Read the model definition and answer for the solid it produces. Units are mm, in the model's axes. Face numbers are marked on the shaded views. A direction names the side the tool comes from. Round coordinates to 2 decimals unless told otherwise and drop trailing zeros. Order: outer loops, then holes, each group sorted by start corner. A loop starts at its lowest first (then second) coordinate and runs counter-clockwise, first axis right, second up. Notation, with made-up numbers: (42, 9) - (59, 9) arc R30 cw to (59, 32) - close; hole circle Ø6 at (-12.5, 55). An arc over 180 degrees is marked (long way). One line per question, with ' | ' between items. Start each with the question number.
1) The part is cut by section C-C, the plane z = -73. Give the vertices of the cut face in (x, y), plus the area to 3 significant figures.
2) Flat-ended cylindrical pins translate along their axes: pin 1 (8 mm diameter, centred on x = 37.5, z = 50.5, fed in from +Y); pin 2 (8 mm diameter, centred on y = 7, z = 38, fed in from +X); pin 3 (6 mm diameter, centred on x = 46, y = 7, fed in from -Z); pin 4 (5 mm diameter, centred on x = 73, z = 0, fed in from -Y). Find the tip coordinate at first contact, or state that the pin passes through.
3) The mould has two halves that part along X. Classify the marked faces 1, 2 and 3: pulls with the +X half, pulls with the -X half, needs draft (parallel to the pull), parting line crosses it, or undercut.
4) The part is cut by section B-B, the plane y = 29.5. Give the vertices of the cut face in (x, z), plus the area to 3 significant figures.
5) The part is cut by section A-A, the plane x = 0. Give the vertices of the cut face in (y, z).
6) The part is cut by section D-D, the plane x = -73. Give the vertices of the cut face in (y, z), plus the area to 3 significant figures.
7) Straight lines are drawn through the part: line 1 (X direction, y = 44, z = 0); line 2 (Y direction, x = 12.5, z = -52). For each, find the intervals that lie inside material, in ascending order. Write a range as from..to.
8) For the marked faces 4 and 5, determine the directions among +Z, -Z, +X, -X, +Y, -Y from which every point of the face is accessible in a straight line to the end or side of a thin tool.
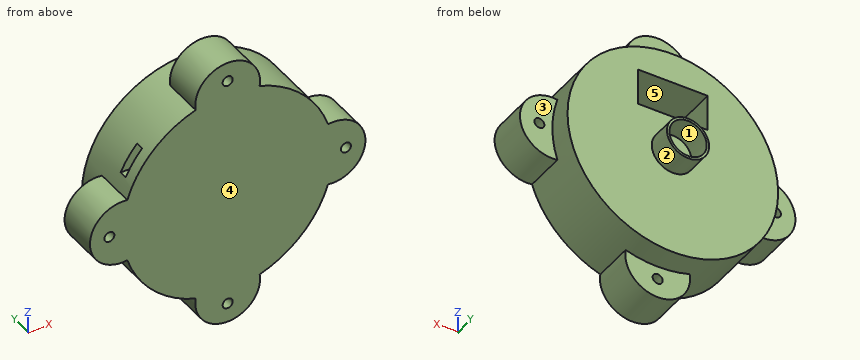
from build123d import *

# Parameters (mm, degrees)
SKETCH2_R           = 65
BOSS_EXTRUDE1_DEPTH = 40
SKETCH4_W           = 43
SKETCH4_H           = 22.5
CUT_EXTRUDE1_DEPTH  = 38
SKETCH6_R           = 3.1
BOSS_EXTRUDE2_DEPTH = 25
SKETCH9_R           = 13
SKETCH9_R_2         = 11.5
BOSS_EXTRUDE3_DEPTH = 15
SKETCH5_W           = 15
SKETCH5_H           = 5
CUT_EXTRUDE2_DEPTH  = 60


with BuildPart() as part:
    # Sketch2 → Boss-Extrude1 (new body)
    with BuildSketch(Plane(origin=(0, 0, 0), x_dir=(1, 0, 0), z_dir=(0, 1, 0))):
        Circle(SKETCH2_R)
    extrude(amount=BOSS_EXTRUDE1_DEPTH)

    # Sketch4 → Cut-Extrude1 (cut)
    with BuildSketch(Plane.XZ.offset(-40)):
        with Locations((0, 35)):
            Rectangle(SKETCH4_W, SKETCH4_H)
    extrude(amount=CUT_EXTRUDE1_DEPTH, mode=Mode.SUBTRACT)

    # Sketch6 → Boss-Extrude2 (add)
    with BuildSketch(Plane(origin=(0, 0, 0), x_dir=(1, 0, 0), z_dir=(0, 1, 0))):
        with BuildLine():
            ThreePointArc((-61.923102255, -19.761816899), (-65, 8.332e-05), (-61.923051591, 19.761975651))
            ThreePointArc((-61.923051591, 19.761975651), (-85, 0.000108957), (-61.923102255, -19.761816899))
        make_face()
        with Locations((-73, 8.332e-05)):
            Circle(SKETCH6_R, mode=Mode.SUBTRACT)
        with BuildLine():
            ThreePointArc((19.761975651, 61.923051591), (0.000108957, 85), (-19.761816899, 61.923102255))
            ThreePointArc((-19.761816899, 61.923102255), (8.332e-05, 65), (19.761975651, 61.923051591))
        make_face()
        with Locations((8.332e-05, 73)):
            Circle(SKETCH6_R, mode=Mode.SUBTRACT)
        with BuildLine():
            ThreePointArc((19.761816899, -61.923102255), (-8.332e-05, -65), (-19.761975651, -61.923051591))
            ThreePointArc((-19.761975651, -61.923051591), (-0.000108957, -85), (19.761816899, -61.923102255))
        make_face()
        with Locations((-8.332e-05, -73)):
            Circle(SKETCH6_R, mode=Mode.SUBTRACT)
        with BuildLine():
            ThreePointArc((61.923051591, -19.761975651), (85, -0.000108957), (61.923102255, 19.761816899))
            ThreePointArc((61.923102255, 19.761816899), (65, -8.332e-05), (61.923051591, -19.761975651))
        make_face()
        with Locations((73, -8.332e-05)):
            Circle(SKETCH6_R, mode=Mode.SUBTRACT)
    extrude(amount=BOSS_EXTRUDE2_DEPTH)

    # Sketch9 → Boss-Extrude3 (add)
    with BuildSketch(Plane(origin=(0, 40, 0), x_dir=(-1, 0, 0), z_dir=(0, -1, 0))):
        Circle(SKETCH9_R)
        Circle(SKETCH9_R_2, mode=Mode.SUBTRACT)
    extrude(amount=-BOSS_EXTRUDE3_DEPTH)

    # Sketch5 → Cut-Extrude2 (cut)
    with BuildSketch(Plane(origin=(-21.5, 0, 62.75), x_dir=(0, 0, 1), z_dir=(-1, 0, 0))):
        with Locations((-26.716652448, 9.82604923)):
            Rectangle(SKETCH5_W, SKETCH5_H)
    extrude(amount=CUT_EXTRUDE2_DEPTH, mode=Mode.SUBTRACT)


solid = part.part
Values:
1) outline: (-18.33, 0) - (-3.1, 0) - (-3.1, 25) - (-18.33, 25) - close; (3.1, 0) - (18.33, 0) - (18.33, 25) - (3.1, 25) - close | area: 762 mm^2
2) pin 1: stops at y = 40 | pin 2: stops at x = 55.4 | pin 3: stops at z = -48.74 | pin 4: passes through
3) face 1: undercut | face 2: parting line crosses it | face 3: needs draft
4) outline: circle Ø130 at (0, 0); hole (-21.5, 23.75) - (21.5, 23.75) - (21.5, 46.25) - (-21.5, 46.25) - close | area: 12,300 mm^2
5) outline: (0, -85) - (25, -85) - (25, -76.1) - (0, -76.1) - close; (0, -69.9) - (25, -69.9) - (25, -65) - (40, -65) - (40, -13) - (55, -13) - (55, -11.5) - (40, -11.5) - (40, 11.5) - (55, 11.5) - (55, 13) - (40, 13) - (40, 23.75) - (2, 23.75) - (2, 46.25) - (40, 46.25) - (40, 65) - (25, 65) - (25, 69.9) - (0, 69.9) - close; (0, 76.1) - (25, 76.1) - (25, 85) - (0, 85) - close
6) outline: (0, -18.33) - (25, -18.33) - (25, -3.1) - (0, -3.1) - close; (0, 3.1) - (25, 3.1) - (25, 18.33) - (0, 18.33) - close | area: 762 mm^2
7) line 1: x = -13..-11.5, 11.5..13 | line 2: y = 0..40
8) face 4: +Z, -Z, +X, -X, -Y | face 5: +Y
